Autodesk Inventor part; units mm, degrees
ref_plane "YZ Plane" through (0, 0, 0) normal (1, 0, 0) x (0, 1, 0)
ref_plane "XZ Plane" through (0, 0, 0) normal (0, 1, 0) x (-1, 0, 0)
ref_plane "XY Plane" through (0, 0, 0) normal (0, 0, 1) x (1, 0, 0)
sketch "Sketch1" plane through (0, 0, 0) normal (0, 0, 1) x (1, 0, 0)
  line L0 (0, 0) -> (600, 0)
  line L1 (600, 0) -> (600, 300)
  line L2 (600, 300) -> (0, 300)
  line L3 (0, 300) -> (0, 0)
  dimension "d0" = 300
  dimension "d1" = 600
extrude "Plate1" add sketch "Sketch1" along normal blind 5
sketch "Sketch2" plane through (595, 0, 5) normal (1, 0, 0) x (0, 1, 0)
  line L0 (300, 0) -> (0, 0)
  line L1 (0, 0) -> (0, -50)
  line L2 (0, -50) -> (300, -50)
  line L3 (300, -50) -> (300, 0)
edge flange "Flange1" height 50 angle 90 thickness 5 bend radius 5 thickness toward (1, 0, 0) relief tear relief width 5 relief depth 2.5 corner gap 5 corner form 2 edges at (600, 150, 0) (0, 150, 0) (300, 0, 0) (300, 300, 0) wall of the first edge with corners at (595, 300, 5) (595, 0, 5) (595, 0, -45) (595, 300, -45)
bend "Bend1"
corner "Corner1"
sketch "Sketch3" plane through (0, 0, 5) normal (0, 0, 1) x (1, 0, 0)
  circle A0 centre (150, 150) radius 32.5
  circle A1 centre (450, 150) radius 32.5
  point P0 (0, 0)
  dimension "d13" = 65
  dimension "d14" = 65
extrude "Extrusion1" cut sketch "Sketch3" against normal blind 10
sketch "Sketch4" plane through (0, 0, 5) normal (0, 0, 1) x (1, 0, 0)
  circle A0 centre (62.5, 260) radius 10
  circle A1 centre (242.5, 260) radius 10
  circle A2 centre (357.5, 260) radius 10
  circle A3 centre (537.5, 260) radius 10
  line L0 (22.5, 236) -> (577.5, 236)
  line L1 (577.5, 304) -> (577.5, 236)
  line L2 (22.5, 304) -> (22.5, 236)
  line L3 (577.5, 304) -> (22.5, 304)
  point P0 (0, 0)
hole "Hole1" at (537.5, 260, 5) at (357.5, 260, 5) at (242.5, 260, 5) at (62.5, 260, 5) direction (0, 0, -1) diameter 20 depth 5 tip angle 118
equation "\"d22\" = Thickness"
equation "\"d3\" = BendReliefWidth"
equation "\"d4\" = BendReliefDepth"
equation "\"d5\" = MinimumRemnant"
equation "\"d6\" = BendRadius"
equation "\"d9\" = BendRadius"
equation "\"d10\" = CornerReliefSize"
equation "\"d11\" = GapSize"
equation "\"d12\" = JacobiRadiusSize"
equation "\"BendRadius\" = Thickness"
equation "\"BendReliefWidth\" = Thickness"
equation "\"BendReliefDepth\" = 0.5 * Thickness"
equation "\"TransitionRadius\" = BendRadius"
equation "\"JacobiRadiusSize\" = BendRadius"
equation "\"GapSize\" = Thickness"
equation "\"d2\" = BendRadius"
properties part number "Side Plate"
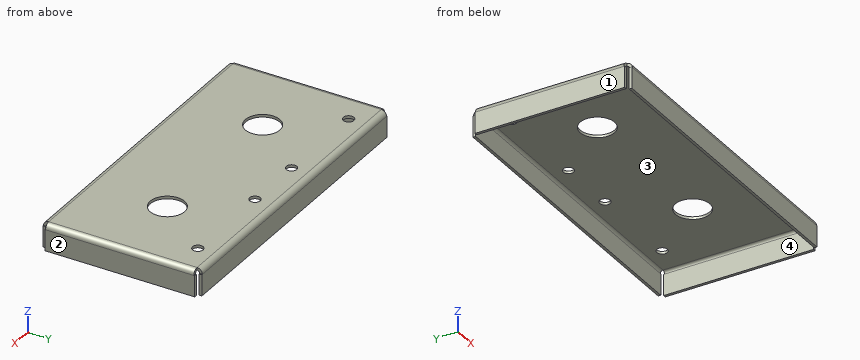
The model under review builds one solid part; all positions refer to its coordinate system, in mm. Face numbers are marked on the shaded views. Round coordinates to 2 decimals unless told otherwise and drop trailing zeros. Write each loop counter-clockwise with the first axis right and the second up, starting at its lowest first coordinate (ties: lowest second). Pieces come first, ordered by that corner, then holes. Notation, with made-up numbers: (35.25, -21.75) - (55.25, -21.75) arc R18 ccw to (55.25, -0.75) - close; hole circle Ø9 at (21, 36). An arc over 180 degrees is marked (long way). Use one line per item in the form item = value.
Q1. For line 1 (X direction, y = 117.5, z = -27); line 2 (Y direction, x = 567.5, z = -19.5); line 3 (X direction, y = 260, z = 1.15), list the stretches that pass through material, from the lowest coordinate up. Write a range as [from, to].
Answer key:
line_1 = [0, 5], [595, 600]
line_2 = [0, 5], [295, 300]
line_3 = [2.11, 52.5], [72.5, 232.5], [252.5, 347.5], [367.5, 527.5], [547.5, 597.89]
Q2. Draft analysis for pull direction X (two halves, no side actions). For the marked faces 1, 2, 3 and 4, state which applies: +X half, -X half, draft (parallel to the pull), parting line (faces both ways), or undercut.
Answer key:
face_1 = -X half
face_2 = +X half
face_3 = undercut
face_4 = undercut
Q3. Consider section D-D (y = 239). State the section outline as (x, z) points.
Answer key:
outline = (0, -45) - (5, -45) - (5, -5) arc R5 cw to (10, 0) - (590, 0) arc R5 cw to (595, -5) - (595, -45) - (600, -45) - (600, -5) arc R10 ccw to (590, 5) - (10, 5) arc R10 ccw to (0, -5) - close
Q4. Insertion check: pin 1 Ø2.5 at (x, z) = (596.5, -17.5) entering from +Y; pin 2 Ø10 at (x, y) = (180.5, 191.5) entering from -Z; pin 3 Ø4 at (x, z) = (3.5, -26.5) entering from -Y. Each pin has a flat end and moves straight along its axis. Give the tip position at first contact, or say it passes through.
Answer key:
pin_1 = 291.46
pin_2 = 0
pin_3 = 8.54
Q5. Consider section C-C (z = -32). State the section outline as (x, y) points, and give its area (3 significant figures).
Answer key:
outline = (0, 8.54) - (5, 8.54) - (5, 291.46) - (0, 291.46) - close; (8.54, 0) - (591.46, 0) - (591.46, 5) - (8.54, 5) - close; (8.54, 295) - (591.46, 295) - (591.46, 300) - (8.54, 300) - close; (595, 8.54) - (600, 8.54) - (600, 291.46) - (595, 291.46) - close
area = 8,660 mm2
Q6. Consider section A-A (y = 150). State the section outline as (x, z) points, and give its area (3 significant figures).
Answer key:
outline = (0, -45) - (5, -45) - (5, -5) arc R5 cw to (10, 0) - (117.5, 0) - (117.5, 5) - (10, 5) arc R10 ccw to (0, -5) - close; (182.5, 0) - (417.5, 0) - (417.5, 5) - (182.5, 5) - close; (482.5, 0) - (590, 0) arc R5 cw to (595, -5) - (595, -45) - (600, -45) - (600, -5) arc R10 ccw to (590, 5) - (482.5, 5) - close
area = 2,770 mm2
Q7. Consider section B-B (x = 242.5). State the section outline as (y, z) points, and give its area (3 significant figures).
Answer key:
outline = (0, -45) - (5, -45) - (5, -5) arc R5 cw to (10, 0) - (250, 0) - (250, 5) - (10, 5) arc R10 ccw to (0, -5) - close; (270, 0) - (290, 0) arc R5 cw to (295, -5) - (295, -45) - (300, -45) - (300, -5) arc R10 ccw to (290, 5) - (270, 5) - close
area = 1,820 mm2
